```python
from build123d import *

# Parameters (mm, degrees)
SKETCH_1_R           = 11
EXTRUDE_1_DEPTH      = 29
SKETCH_2_OUTSIDE_W   = 32.506
SKETCH_2_OUTSIDE_H   = 32.506
SKETCH_2_OUTSIDE_R   = 10
CUT_EXTRUDE_1_DEPTH  = 9
SKETCH_3_R           = 7.7
CUT_EXTRUDE_2_DEPTH  = 20
SKETCH_4_R           = 2.1
CUT_EXTRUDE_3_DEPTH  = 25
CHAMFER_1_SIZE       = 3
EXTRUDE_START        = 10
SKETCH_5_R           = 10
EXTRUDE_2_DEPTH      = 10
CUT_EXTRUDE_5_DEPTH  = 19
CUT_EXTRUDE_6_DEPTH  = 19
CHAMFER_2_SIZE       = 0.4
SKETCH_12_R          = 10
CUT_EXTRUDE_9_DEPTH  = 10
SKETCH_13_R          = 4.1
CUT_EXTRUDE_10_DEPTH = 9
CHAMFER_3_SIZE       = 0.4
SKETCH_15_R          = 4.1
EXTRUDE_3_DEPTH      = 9
SKETCH_16_R          = 6
EXTRUDE_4_DEPTH      = 70
CHAMFER_4_SIZE       = 1
SKETCH_17_R          = 2.05
CUT_EXTRUDE_12_DEPTH = 35


with BuildPart() as part:
    # 草图1 → 凸台-拉伸1 (new body)
    with BuildSketch(Plane.XY):
        with Locations(Location((0, 0, 0), (0, 0, 180))):
            Circle(SKETCH_1_R)
    extrude(amount=EXTRUDE_1_DEPTH)

    # 草图2 outside → 切除-拉伸1 (cut)
    with BuildSketch(Plane.XY.offset(29)):
        Rectangle(SKETCH_2_OUTSIDE_W, SKETCH_2_OUTSIDE_H)
        Circle(SKETCH_2_OUTSIDE_R, mode=Mode.SUBTRACT)
    extrude(amount=-CUT_EXTRUDE_1_DEPTH, mode=Mode.SUBTRACT)

    # 草图3 → 切除-拉伸2 (cut)
    with BuildSketch(Plane(origin=(0, 0, 0), x_dir=(-1, 0, 0), z_dir=(0, 0, -1))):
        Circle(SKETCH_3_R)
    extrude(amount=-CUT_EXTRUDE_2_DEPTH, mode=Mode.SUBTRACT)

    # 草图4 → 切除-拉伸3 (cut, symmetric)
    with BuildSketch(Plane(origin=(0, 0, 0), x_dir=(1, 0, 0), z_dir=(0, 1, 0))):
        with BuildLine():
            Line((-2.1, 0), (-2.1, -17))
            ThreePointArc((-2.1, -17), (0, -14.9), (2.1, -17))
            Line((2.1, -17), (2.1, 0))
            Line((2.1, 0), (-2.1, 0))
        make_face()
        with Locations((0, -17)):
            Circle(SKETCH_4_R)
    extrude(amount=CUT_EXTRUDE_3_DEPTH, both=True, mode=Mode.SUBTRACT)

    # 倒角1
    chamfer_1_edges = [part.edges().sort_by_distance(p)[0] for p in [
        (7.7, 0, 0),
        (-6.142475071, -4.643274706, 0),
    ]]
    chamfer(chamfer_1_edges, length=CHAMFER_1_SIZE)

    # 草图5 → 凸台-拉伸2 (add)
    with BuildSketch(Plane.XY.offset(29).offset(EXTRUDE_START)):
        Circle(SKETCH_5_R)
    extrude(amount=-EXTRUDE_2_DEPTH)

    # 草图6 → 切除-拉伸5 (cut)
    with BuildSketch(Plane.XY.offset(39)):
        with BuildLine():
            Line((3.122498999, 2.5), (-3.122498999, 2.5))
            ThreePointArc((-3.122498999, 2.5), (-1.324764885, -3.774254628), (4, 0))
            ThreePointArc((4, 0), (3.774254628, 1.324764885), (3.122498999, 2.5))
        make_face()
    extrude(amount=-CUT_EXTRUDE_5_DEPTH, mode=Mode.SUBTRACT)

    # 草图7 → 切除-拉伸6 (cut)
    with BuildSketch(Plane.XY.offset(39)):
        with BuildLine():
            Line((3.170173497, 2.6), (-3.170173497, 2.6))
            ThreePointArc((-3.170173497, 2.6), (0, -4.1), (3.170173497, 2.6))
        make_face()
    extrude(amount=-CUT_EXTRUDE_6_DEPTH, mode=Mode.SUBTRACT)

    # 倒角2
    chamfer_2_edges = [part.edges().sort_by_distance(p)[0] for p in [
        (0, -4.1, 39),
        (0, 2.6, 39),
    ]]
    chamfer(chamfer_2_edges, length=CHAMFER_2_SIZE)

    # 草图12 → 切除-拉伸9 (cut)
    with BuildSketch(Plane.XY.offset(39)):
        Circle(SKETCH_12_R)
    extrude(amount=-CUT_EXTRUDE_9_DEPTH, mode=Mode.SUBTRACT)

    # 草图13 → 切除-拉伸10 (cut)
    with BuildSketch(Plane.XY.offset(29)):
        Circle(SKETCH_13_R)
    extrude(amount=-CUT_EXTRUDE_10_DEPTH, mode=Mode.SUBTRACT)

    # 倒角3
    chamfer_3_edges = [part.edges().sort_by_distance(p)[0] for p in [
        (-10, 0, 29),
    ]]
    chamfer(chamfer_3_edges, length=CHAMFER_3_SIZE)

    # 草图15 → 凸台-拉伸3 (add)
    with BuildSketch(Plane.XY.offset(29)):
        Circle(SKETCH_15_R)
    extrude(amount=-EXTRUDE_3_DEPTH)

    # 草图16 → 凸台-拉伸4 (add)
    with BuildSketch(Plane.XY.offset(29)):
        Circle(SKETCH_16_R)
    extrude(amount=EXTRUDE_4_DEPTH)

    # 倒角4
    chamfer_4_edges = [part.edges().sort_by_distance(p)[0] for p in [
        (-6, 0, 99),
    ]]
    chamfer(chamfer_4_edges, length=CHAMFER_4_SIZE)

    # 草图17 → 切除-拉伸12 (cut, symmetric)
    with BuildSketch(Plane(origin=(0, 0, 0), x_dir=(1, 0, 0), z_dir=(0, 1, 0))):
        with Locations(Location((0, -61.5, 0), (0, 0, 270))):
            Circle(SKETCH_17_R)
    extrude(amount=CUT_EXTRUDE_12_DEPTH, both=True, mode=Mode.SUBTRACT)


solid = part.part
```
Design review of the part built by this model. Coordinates are the model's own, in mm. A direction names the side the tool comes from. Round coordinates to 2 decimals unless told otherwise and drop trailing zeros. Write each loop counter-clockwise with the first axis right and the second up, starting at its lowest first coordinate (ties: lowest second). Pieces come first, ordered by that corner, then holes. Notation, with made-up numbers: (-19, 12) -> (38, 12) arc R14 ccw to (38, 25) -> close; hole circle Ø8 at (20, 0.25). An arc over 180 degrees is marked (long way). Answer in a Markdown table with one row per item.
Q1. Draft analysis for pull direction Y (two halves, no side actions). For faces 1 (the face through (7.844, 0.151, 2.854)), 2 (the face through (-2.17, -9.76, 24.36)), 3 (the face through (-2.1, 9, 8)), state which applies: +Y half, -Y half, draft (parallel to the pull), parting line (faces both ways), or undercut.
The answers:
| item | result |
|---|---|
| face 1 | undercut |
| face 2 | parting line |
| face 3 | draft |
Q2. Clearance check with flat-ended pins moving along their axes: pin 1 Ø8 at (x, y) = (-6.5, 2.5) entering from -Z; pin 2 Ø6 at (y, z) = (0.5, 39.5) entering from -X; pin 3 Ø3 at (y, z) = (3, 83) entering from -X; pin 4 Ø12 at (x, z) = (1, 28) entering from +Y. State where each tip first meets the part, or that it passes through.
The answers:
| item | result |
|---|---|
| pin 1 | z = 0 |
| pin 2 | x = -6 |
| pin 3 | x = -5.81 |
| pin 4 | y = 10 |
Q3. Take a section at B-B, the plane x = 0. State the section outline as (y, z) points.
The answers:
| item | result |
|---|---|
| outline | (-11, 19.1) -> (-7.7, 19.1) -> (-7.7, 20) -> (7.7, 20) -> (7.7, 19.1) -> (11, 19.1) -> (11, 20) -> (10, 20) -> (10, 28.6) -> (9.6, 29) -> (6, 29) -> (6, 59.45) -> (-6, 59.45) -> (-6, 29) -> (-9.6, 29) -> (-10, 28.6) -> (-10, 20) -> (-11, 20) -> close; (-6, 63.55) -> (6, 63.55) -> (6, 98) -> (5, 99) -> (-5, 99) -> (-6, 98) -> close |
Q4. Take a section at D-D, the plane z = 22. State the section outline as (x, y) points.
The answers:
| item | result |
|---|---|
| outline | circle Ø20 at (0, 0) |
Q5. For faces 4 (the face through (-7.844, -0.151, 2.854)), 5 (the face through (2.1, 9, 9)), 6 (the face through (0, 0, 99)), 7 (the face through (2.38, 10.74, 9.86)), 8 (the face through (5.54, -2.3, 63.02)), list the 3-axis set-ups (+Z, -Z, +X, -X, +Y, -Y) from which the entire face can be reached by the end or side of a thin tool; tool diameter is ignored.
The answers:
| item | result |
|---|---|
| face 4 | -Z |
| face 5 | -Z, +Y, -Y |
| face 6 | +Z, +X, -X, +Y, -Y |
| face 7 | +Z, -Z |
| face 8 | +Z |
Q6. Take a section at C-C, the plane z = 53. State the section outline as (x, y) points, then the cut area to 3 significant figures.
The answers:
| item | result |
|---|---|
| outline | circle Ø12 at (0, 0) |
| area | 113 mm² |
Q7. To check wall thickness, follow L1, parallel to X at y = -0.25, z = 61.5; L2, parallel to Z at x = 0, y = 0.5; L3, parallel to Z at x = -7, y = 3. State the ranges of each line that lie inside material, in increasing order. Write a range as [from, to].
The answers:
| item | result |
|---|---|
| L1 | [-5.99, -2.05], [2.05, 5.99] |
| L2 | [20, 59.45], [63.55, 99] |
| L3 | [20, 29] |
Q8. Take a section at A-A, the plane y = 0. State the section outline as (x, z) points.
The answers:
| item | result |
|---|---|
| outline | (-11, 0) -> (-10.7, 0) -> (-7.7, 3) -> (-7.7, 20) -> (7.7, 20) -> (7.7, 3) -> (10.7, 0) -> (11, 0) -> (11, 20) -> (10, 20) -> (10, 28.6) -> (9.6, 29) -> (6, 29) -> (6, 98) -> (5, 99) -> (-5, 99) -> (-6, 98) -> (-6, 29) -> (-9.6, 29) -> (-10, 28.6) -> (-10, 20) -> (-11, 20) -> close; hole circle Ø4.1 at (0, 61.5) |
